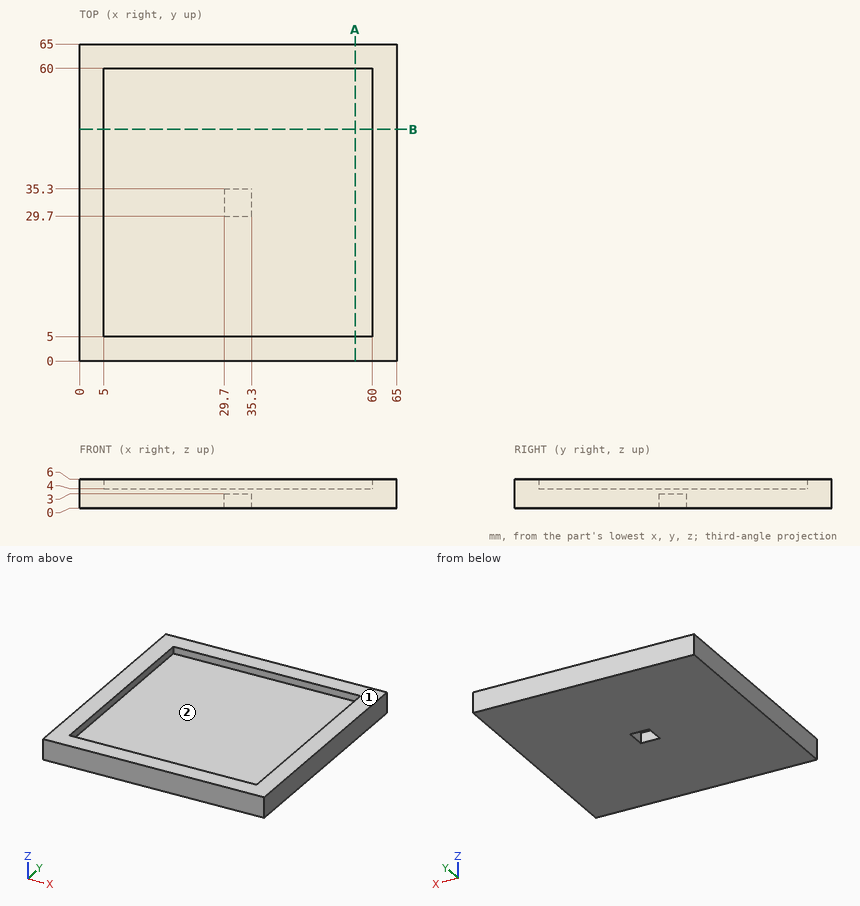
For this review, use the dimensioned drawing (mm, ordinates from the lowest corner) and the shaded views. Round coordinates to 2 decimals unless told otherwise and drop trailing zeros. Order: outer loops, then holes, each group sorted by start corner. A loop starts at its lowest first (then second) coordinate and runs counter-clockwise, first axis right, second up. Notation, with made-up numbers: (51, 10) - (87, 10) arc R24 ccw to (87, 31) - close; hole circle Ø3 at (-38.75, -17.75). An arc over 180 degrees is marked (long way). Use one line per item in the form item = value.
Q1. Add section A-A on x = 56.5. Give the boundary of the cut face in (y, z), then the cut area to 3 significant figures.
Response values:
outline = (0, 0) - (65, 0) - (65, 6) - (60, 6) - (60, 4) - (5, 4) - (5, 6) - (0, 6) - close
area = 280 mm^2
Q2. Mouldability with a two-part tool opening along X and no side actions: class the marked faces 1 and 2 as pulls with the +X half, pulls with the -X half, needs draft (parallel to the pull), parting line crosses it, or undercut.
Response values:
face_1 = needs draft
face_2 = undercut
Q3. Clearance check with flat-ended pins moving along their axes: P1, Ø10, axis at x = 29.5, y = 15, coming from the +Z side; P2, Ø3, axis at x = 32.5, y = 32.5, coming from the -Z side. State where each tip first meets the part, or that it passes through.
Response values:
P1 = 4
P2 = 3
Q4. To check wall thickness, follow line 1 (Y direction, x = 37.5, z = 5.1); line 2 (Z direction, x = 15, y = 18). State the ranges of each line that lie inside material, in increasing order.
Response values:
line_1 = 0 to 5, 60 to 65
line_2 = 0 to 4
